Verification items for the finished model (mm, model axes). Face numbers are marked on the shaded views. A direction names the side the tool comes from. Give positions to 0.01 mm unless a question says otherwise; leave off trailing zeros. Loops run counter-clockwise (first coordinate to the right, second up) from the corner with the lowest first, then second, coordinate; pieces in that order, holes last. Notation, with made-up numbers: M 68.25,54 L 80.25,54 A16 ccw 80.25,62 Z; hole C -21.75,47 d4. An arc over 180 degrees is marked long. Answer in a Markdown table with one row per item.
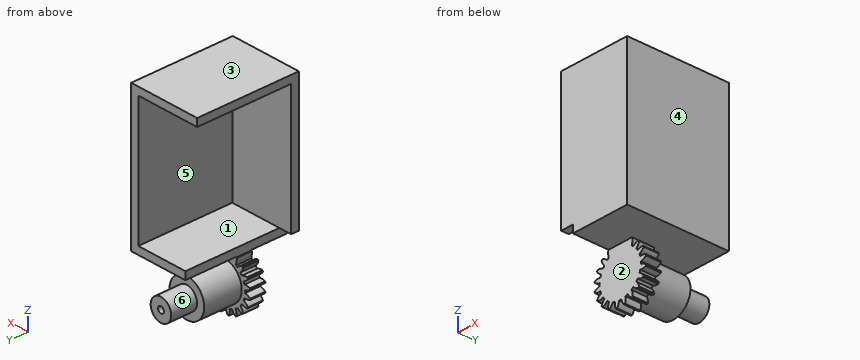
```python
from build123d import *

# Parameters (mm, degrees)
EXTRUDE_1_DEPTH = 6
EXTRUDE_2_DEPTH = 20
SKETCH_3_W      = 25
SKETCH_3_H      = 50
EXTRUDE_3_DEPTH = 3
EXTRUDE_4_DEPTH = 6
SKETCH_5_R      = 7.35
EXTRUDE_5_DEPTH = 14.8
SKETCH_6_R      = 4.35
SKETCH_6_R_2    = 1.25
EXTRUDE_6_DEPTH = 10.2


with BuildPart() as part:
    # 草图1 → 凸台-拉伸1 (new body)
    with BuildSketch(Plane(origin=(0, 0, 0), x_dir=(1, 0, 0), z_dir=(0, 1, 0))):
        with BuildLine():
            Line((-5, 0), (-5, -13))
            Line((-5, -13), (15, -13))
            Line((15, -13), (15, -63))
            Line((15, -63), (-10, -63))
            Line((-10, -63), (-10, -66))
            Line((-10, -66), (18, -66))
            Line((18, -66), (18, -10))
            Line((18, -10), (5, -10))
            Line((5, -10), (5, 0))
            ThreePointArc((5, 0), (0, 5), (-5, 0))
        make_face()
    extrude(amount=-EXTRUDE_1_DEPTH)

    # 草图2 → 凸台-拉伸2 (add, symmetric)
    with BuildSketch(Plane(origin=(0, 0, 0), x_dir=(1, 0, 0), z_dir=(0, 1, 0))):
        Polygon((-5, -13), (15, -13), (15, -63), (-10, -63), (-10, -66), (18, -66), (18, -10), (-5, -10), align=None)
    extrude(amount=EXTRUDE_2_DEPTH, both=True)

    # 草图3 → 凸台-拉伸3 (add)
    with BuildSketch(Plane.XZ.offset(20)):
        with Locations((2.5, 38)):
            Rectangle(SKETCH_3_W, SKETCH_3_H)
    extrude(amount=-EXTRUDE_3_DEPTH)

    # 草图4 → 凸台-拉伸4 (add)
    with BuildSketch(Plane.XZ.offset(6)):
        with BuildLine():
            ThreePointArc((-0.504732798, 8.734428762), (-0.823506466, 9.891100464), (-1.470958285, 10.901205517))
            ThreePointArc((-1.470958285, 10.901205517), (-1.726760313, 10.86362273), (-1.981608382, 10.820038273))
            ThreePointArc((-1.981608382, 10.820038273), (-2.283953757, 9.65896405), (-2.228374617, 8.460457882))
            ThreePointArc((-2.228374617, 8.460457882), (-2.708170263, 8.319303747), (-3.17911634, 8.150964378))
            ThreePointArc((-3.17911634, 8.150964378), (-3.839719327, 9.152518056), (-4.767622226, 9.913111434))
            ThreePointArc((-4.767622226, 9.913111434), (-4.999290692, 9.798320906), (-5.228197271, 9.678117239))
            ThreePointArc((-5.228197271, 9.678117239), (-5.156953143, 8.480440175), (-4.733735466, 7.357767973))
            ThreePointArc((-4.733735466, 7.357767973), (-5.146429214, 7.075257405), (-5.542305825, 6.76962681))
            ThreePointArc((-5.542305825, 6.76962681), (-6.480073708, 7.518023412), (-7.597598086, 7.954652936))
            ThreePointArc((-7.597598086, 7.954652936), (-7.782455665, 7.773891163), (-7.963013783, 7.588834659))
            ThreePointArc((-7.963013783, 7.588834659), (-7.525154025, 6.471791729), (-6.775725305, 5.53484847))
            ThreePointArc((-6.775725305, 5.53484847), (-7.080919818, 5.138635571), (-7.3629758, 4.725631002))
            ThreePointArc((-7.3629758, 4.725631002), (-8.486113324, 5.147612255), (-9.683868109, 5.217537585))
            ThreePointArc((-9.683868109, 5.217537585), (-9.803819655, 4.988498789), (-9.918355025, 4.756704069))
            ThreePointArc((-9.918355025, 4.756704069), (-9.1567404, 3.829639217), (-8.154459943, 3.170139435))
            ThreePointArc((-8.154459943, 3.170139435), (-8.322280653, 2.699008286), (-8.462906403, 2.219057507))
            ThreePointArc((-8.462906403, 2.219057507), (-9.661473042, 2.273316945), (-10.82221365, 1.969693302))
            ThreePointArc((-10.82221365, 1.969693302), (-10.86551747, 1.714797397), (-10.902818572, 1.458954141))
            ThreePointArc((-10.902818572, 1.458954141), (-9.892001226, 0.812614936), (-8.734979226, 0.495115065))
            ThreePointArc((-8.734979226, 0.495115065), (-8.748998674, -0.004816736), (-8.734428762, -0.504732798))
            ThreePointArc((-8.734428762, -0.504732798), (-9.891100464, -0.823506466), (-10.901205517, -1.470958285))
            ThreePointArc((-10.901205517, -1.470958285), (-10.86362273, -1.726760313), (-10.820038273, -1.981608382))
            ThreePointArc((-10.820038273, -1.981608382), (-9.65896405, -2.283953757), (-8.460457882, -2.228374617))
            ThreePointArc((-8.460457882, -2.228374617), (-8.319303747, -2.708170263), (-8.150964378, -3.17911634))
            ThreePointArc((-8.150964378, -3.17911634), (-9.152518056, -3.839719327), (-9.913111434, -4.767622226))
            ThreePointArc((-9.913111434, -4.767622226), (-9.798320906, -4.999290692), (-9.678117239, -5.228197271))
            ThreePointArc((-9.678117239, -5.228197271), (-8.480440175, -5.156953143), (-7.357767973, -4.733735466))
            ThreePointArc((-7.357767973, -4.733735466), (-7.075257405, -5.146429214), (-6.76962681, -5.542305825))
            ThreePointArc((-6.76962681, -5.542305825), (-7.518023412, -6.480073708), (-7.954652936, -7.597598086))
            ThreePointArc((-7.954652936, -7.597598086), (-7.773891163, -7.782455665), (-7.588834659, -7.963013783))
            ThreePointArc((-7.588834659, -7.963013783), (-6.471791729, -7.525154025), (-5.53484847, -6.775725305))
            ThreePointArc((-5.53484847, -6.775725305), (-5.138635571, -7.080919818), (-4.725631002, -7.3629758))
            ThreePointArc((-4.725631002, -7.3629758), (-5.147612255, -8.486113324), (-5.217537585, -9.683868109))
            ThreePointArc((-5.217537585, -9.683868109), (-4.988498789, -9.803819655), (-4.756704069, -9.918355025))
            ThreePointArc((-4.756704069, -9.918355025), (-3.829639217, -9.1567404), (-3.170139435, -8.154459943))
            ThreePointArc((-3.170139435, -8.154459943), (-2.699008286, -8.322280653), (-2.219057507, -8.462906403))
            ThreePointArc((-2.219057507, -8.462906403), (-2.273316945, -9.661473042), (-1.969693302, -10.82221365))
            ThreePointArc((-1.969693302, -10.82221365), (-1.714797397, -10.86551747), (-1.458954141, -10.902818572))
            ThreePointArc((-1.458954141, -10.902818572), (-0.812614936, -9.892001226), (-0.495115065, -8.734979226))
            ThreePointArc((-0.495115065, -8.734979226), (0.004816736, -8.748998674), (0.504732798, -8.734428762))
            ThreePointArc((0.504732798, -8.734428762), (0.823506466, -9.891100464), (1.470958285, -10.901205517))
            ThreePointArc((1.470958285, -10.901205517), (1.726760313, -10.86362273), (1.981608382, -10.820038273))
            ThreePointArc((1.981608382, -10.820038273), (2.283953757, -9.65896405), (2.228374617, -8.460457882))
            ThreePointArc((2.228374617, -8.460457882), (2.708170263, -8.319303747), (3.17911634, -8.150964378))
            ThreePointArc((3.17911634, -8.150964378), (3.839719327, -9.152518056), (4.767622226, -9.913111434))
            ThreePointArc((4.767622226, -9.913111434), (4.999290692, -9.798320906), (5.228197271, -9.678117239))
            ThreePointArc((5.228197271, -9.678117239), (5.156953143, -8.480440175), (4.733735466, -7.357767973))
            ThreePointArc((4.733735466, -7.357767973), (5.146429214, -7.075257405), (5.542305825, -6.76962681))
            ThreePointArc((5.542305825, -6.76962681), (6.480073708, -7.518023412), (7.597598086, -7.954652936))
            ThreePointArc((7.597598086, -7.954652936), (7.782455665, -7.773891163), (7.963013783, -7.588834659))
            ThreePointArc((7.963013783, -7.588834659), (7.525154025, -6.471791729), (6.775725305, -5.53484847))
            ThreePointArc((6.775725305, -5.53484847), (7.080919818, -5.138635571), (7.3629758, -4.725631002))
            ThreePointArc((7.3629758, -4.725631002), (8.486113324, -5.147612255), (9.683868109, -5.217537585))
            ThreePointArc((9.683868109, -5.217537585), (9.803819655, -4.988498789), (9.918355025, -4.756704069))
            ThreePointArc((9.918355025, -4.756704069), (9.1567404, -3.829639217), (8.154459943, -3.170139435))
            ThreePointArc((8.154459943, -3.170139435), (8.322280653, -2.699008286), (8.462906403, -2.219057507))
            ThreePointArc((8.462906403, -2.219057507), (9.661473042, -2.273316945), (10.82221365, -1.969693302))
            ThreePointArc((10.82221365, -1.969693302), (10.86551747, -1.714797397), (10.902818572, -1.458954141))
            ThreePointArc((10.902818572, -1.458954141), (9.892001226, -0.812614936), (8.734979226, -0.495115065))
            ThreePointArc((8.734979226, -0.495115065), (8.748998674, 0.004816736), (8.734428762, 0.504732798))
            ThreePointArc((8.734428762, 0.504732798), (9.891100464, 0.823506466), (10.901205517, 1.470958285))
            ThreePointArc((10.901205517, 1.470958285), (10.86362273, 1.726760313), (10.820038273, 1.981608382))
            ThreePointArc((10.820038273, 1.981608382), (9.65896405, 2.283953757), (8.460457882, 2.228374617))
            ThreePointArc((8.460457882, 2.228374617), (8.319303747, 2.708170263), (8.150964378, 3.17911634))
            ThreePointArc((8.150964378, 3.17911634), (9.152518056, 3.839719327), (9.913111434, 4.767622226))
            ThreePointArc((9.913111434, 4.767622226), (9.798320906, 4.999290692), (9.678117239, 5.228197271))
            ThreePointArc((9.678117239, 5.228197271), (8.480440175, 5.156953143), (7.357767973, 4.733735466))
            ThreePointArc((7.357767973, 4.733735466), (7.075257405, 5.146429214), (6.76962681, 5.542305825))
            ThreePointArc((6.76962681, 5.542305825), (7.518023412, 6.480073708), (7.954652936, 7.597598086))
            ThreePointArc((7.954652936, 7.597598086), (7.773891163, 7.782455665), (7.588834659, 7.963013783))
            ThreePointArc((7.588834659, 7.963013783), (6.471791729, 7.525154025), (5.53484847, 6.775725305))
            ThreePointArc((5.53484847, 6.775725305), (5.138635571, 7.080919818), (4.725631002, 7.3629758))
            ThreePointArc((4.725631002, 7.3629758), (5.147612255, 8.486113324), (5.217537585, 9.683868109))
            ThreePointArc((5.217537585, 9.683868109), (4.988498789, 9.803819655), (4.756704069, 9.918355025))
            ThreePointArc((4.756704069, 9.918355025), (3.829639217, 9.1567404), (3.170139435, 8.154459943))
            ThreePointArc((3.170139435, 8.154459943), (2.699008286, 8.322280653), (2.219057507, 8.462906403))
            ThreePointArc((2.219057507, 8.462906403), (2.273316945, 9.661473042), (1.969693302, 10.82221365))
            ThreePointArc((1.969693302, 10.82221365), (1.714797397, 10.86551747), (1.458954141, 10.902818572))
            ThreePointArc((1.458954141, 10.902818572), (0.812614936, 9.892001226), (0.495115065, 8.734979226))
            ThreePointArc((0.495115065, 8.734979226), (-0.004816736, 8.748998674), (-0.504732798, 8.734428762))
        make_face()
    extrude(amount=-EXTRUDE_4_DEPTH)

    # 草图5 → 凸台-拉伸5 (add)
    with BuildSketch(Plane(origin=(0, 0, 0), x_dir=(1, 0, 0), z_dir=(0, 1, 0))):
        with Locations(Location((0, 0, 0), (0, 0, 270))):
            Circle(SKETCH_5_R)
    extrude(amount=EXTRUDE_5_DEPTH)

    # 草图6 → 凸台-拉伸6 (add)
    with BuildSketch(Plane(origin=(0, 14.8, 0), x_dir=(1, 0, 0), z_dir=(0, 1, 0))):
        with Locations(Location((0, 0, 0), (0, 0, 270))):
            Circle(SKETCH_6_R)
        with Locations(Location((0, 0, 0), (0, 0, 270))):
            Circle(SKETCH_6_R_2, mode=Mode.SUBTRACT)
    extrude(amount=EXTRUDE_6_DEPTH)


solid = part.part
```
Item 1: Release check for a two-part mould opening along Z. For the marked faces 1, 2 and 3 record: released by +Z, released by -Z, zero draft, split by the parting line, or undercut.
Reported:
| item | result |
|---|---|
| face 1 | undercut |
| face 2 | zero draft |
| face 3 | released by +Z |
Item 2: Go/stop test with flat-tipped pins: pin 1 (6 mm diameter, centred on y = 8.5, z = 46, fed in from -X); pin 2 (2 mm diameter, centred on x = 13.5, y = 12, fed in from -Z); pin 3 (1.5 mm diameter, centred on x = -0.5, y = 12, fed in from -Z). Record where each tip stops, or that it passes through.
Reported:
| item | result |
|---|---|
| pin 1 | stops at x = 15 |
| pin 2 | stops at z = 10 |
| pin 3 | stops at z = -7.35 |
Item 3: Tool access check on the marked faces 4, 5 and 6. Record the directions out of +Z, -Z, +X, -X, +Y, -Y that give a thin tool (end or side, any length) a straight path to the whole face; none if there is none.
Reported:
| item | result |
|---|---|
| face 4 | +Z, -Z, +X, +Y, -Y |
| face 5 | -X, +Y |
| face 6 | +Y |
Item 4: Sectioned sample at A-A (y = 3). Record the cut outline in (x, z).
Reported:
| item | result |
|---|---|
| outline | M -10,63 L 15,63 L 15,13 L -5,13 L -5,10 L 18,10 L 18,66 L -10,66 Z; C 0,0 d14.7 |
Item 5: Sectioned sample at B-B (x = 14.25). Record the cut outline in (y, z), and give its area (3 significant figures).
Reported:
| item | result |
|---|---|
| outline | M -20,10 L 20,10 L 20,13 L -17,13 L -17,63 L 20,63 L 20,66 L -20,66 Z |
| area | 390 mm^2 |
Item 6: Sectioned sample at D-D (z = 12). Record the cut outline in (x, y), and give its area (3 significant figures).
Reported:
| item | result |
|---|---|
| outline | M -5,-20 L 18,-20 L 18,20 L -5,20 Z |
| area | 920 mm^2 |
Item 7: Scan lines: L1, parallel to X at y = 20, z = 0; L2, parallel to Z at x = 14, y = -9.5; L3, parallel to Z at x = 1, y = 14.5. Record each from-to range of solid material in increasing order. Write a range as [from, to].
Reported:
| item | result |
|---|---|
| L1 | x = [-4.35, -1.25], [1.25, 4.35] |
| L2 | z = [10, 13], [63, 66] |
| L3 | z = [-7.28, 7.28], [10, 13], [63, 66] |
Item 8: Sectioned sample at C-C (z = 23.5). Record the cut outline in (x, y), and give its area (3 significant figures).
Reported:
| item | result |
|---|---|
| outline | M -10,-20 L 18,-20 L 18,20 L 15,20 L 15,-17 L -10,-17 Z |
| area | 195 mm^2 |
